Input: part model. Units: mm. Frame: model coordinates. Face numbers are marked on the shaded views. Give positions to 0.01 mm unless a question says otherwise; leave off trailing zeros. Write each loop counter-clockwise with the first axis right and the second up, starting at its lowest first coordinate (ties: lowest second). Pieces come first, ordered by that corner, then holes. Notation, with made-up numbers: (71, -40) - (117, -40) arc R7 cw to (117, -29) - close; hole circle Ø9 at (-9, 73). An arc over 180 degrees is marked (long way). Use a Markdown table: item, result. Add a question column.
1. Section query A-A, the plane z = 3.05. Return loops of the section in (x, y), plus the area to 3 significant figures.
2. Material intervals for probe 1 along Z at (x, y) = (1.25, 4); probe 2 along Y at (x, z) = (-1.5, 1.05); probe 3 along X at (y, z) = (-2.25, 1.7), sorted ascending.
3. Pin query (flat end, axial travel): pin 1 (1.5 mm diameter, centred on y = -3.5, z = 1.5, fed in from -X); pin 2 (1.5 mm diameter, centred on x = 1, z = 1, fed in from -Y). Return the tip coordinate at first contact, or that it passes through.
4. Section query B-B, the plane y = 0. Return loops of the section in (x, z).
5. Section query C-C, the plane y = 2. Return loops of the section in (x, z), plus the area to 3 significant figures.
6. Mould query, pull axis Y, two halves, no side actions, for the marked faces 1, 2 and 3. Classes: released by +Y, released by -Y, zero draft, split by the parting line, or undercut.
7. Section query D-D, the plane z = 0.5. Return loops of the section in (x, y), plus the area to 3 significant figures.
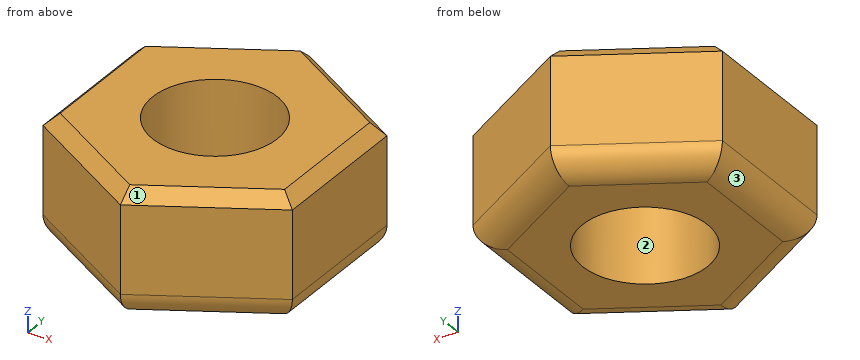
```python
from build123d import *

# Parameters (mm, degrees)
F0_R     = 2.5
F1_DEPTH = 5
F2_R     = 1
F3_SIZE  = 0.5


with BuildPart() as f1:
    # F0 (on Top) → F1 (new body)
    with BuildSketch(Plane.XY):
        Polygon((5, -2.886751), (5, 2.886751), (0, 5.773503), (-5, 2.886751), (-5, -2.886751), (0, -5.773503), align=None)
        Circle(F0_R, mode=Mode.SUBTRACT)
    extrude(amount=F1_DEPTH)

    # F2
    f2_edges = [f1.edges().sort_by_distance(p)[0] for p in [
        (-2.5, -4.330127, 0),
        (2.5, -4.330127, 0),
        (5, 0, 0),
        (2.5, 4.330127, 0),
        (-2.5, 4.330127, 0),
        (-5, 0, 0),
    ]]
    fillet(f2_edges, radius=F2_R)

    # F3
    f3_edges = [f1.edges().sort_by_distance(p)[0] for p in [
        (-2.5, -4.330127, 5),
        (2.5, -4.330127, 5),
        (5, 0, 5),
        (2.5, 4.330127, 5),
        (-2.5, 4.330127, 5),
        (-5, 0, 5),
    ]]
    chamfer(f3_edges, length=F3_SIZE)


solid = f1.part
```
Result sheet:
| question | item | result |
|---|---|---|
| 1 | outline | (-5, -2.89) - (0, -5.77) - (5, -2.89) - (5, 2.89) - (0, 5.77) - (-5, 2.89) - close; hole circle Ø5 at (0, 0) |
| 1 | area | 67.0 mm² |
| 2 | probe 1 | z = 0 to 5 |
| 2 | probe 2 | y = -4.91 to -2, 2 to 4.91 |
| 2 | probe 3 | x = -5 to -1.09, 1.09 to 5 |
| 3 | pin 1 | stops at x = -5 |
| 3 | pin 2 | stops at y = -5.63 |
| 4 | outline | (-5, 1) arc R1 ccw to (-4, 0) - (-2.5, 0) - (-2.5, 5) - (-4.5, 5) - (-5, 4.5) - close; (2.5, 0) - (4, 0) arc R1 ccw to (5, 1) - (5, 4.5) - (4.5, 5) - (2.5, 5) - close |
| 5 | outline | (-5, 1) arc R1 ccw to (-4, 0) - (-1.5, 0) - (-1.5, 5) - (-4.5, 5) - (-5, 4.5) - close; (1.5, 0) - (4, 0) arc R1 ccw to (5, 1) - (5, 4.5) - (4.5, 5) - (1.5, 5) - close |
| 5 | area | 34.3 mm² |
| 6 | face 1 | released by -Y |
| 6 | face 2 | undercut |
| 6 | face 3 | zero draft |
| 7 | outline | (-4.87, -2.81) - (0, -5.62) - (4.87, -2.81) - (4.87, 2.81) - (0, 5.62) - (-4.87, 2.81) - close; hole circle Ø5 at (0, 0) |
| 7 | area | 62.4 mm² |
